Check sheet for the drawn part. Datum: minimum x, y, z corner. Units: mm. Give positions to 0.01 mm unless a question says otherwise; leave off trailing zeros. Loops run counter-clockwise (first coordinate to the right, second up) from the corner with the lowest first, then second, coordinate; pieces in that order, holes last. Notation, with made-up numbers: (-31.5, 0.25) - (-15.5, 0.25) arc R30 cw to (-15.5, 30.25) - close; hole circle Ø11 at (75, -24.75). An arc over 180 degrees is marked (long way). Use one line per item in the form item = value.
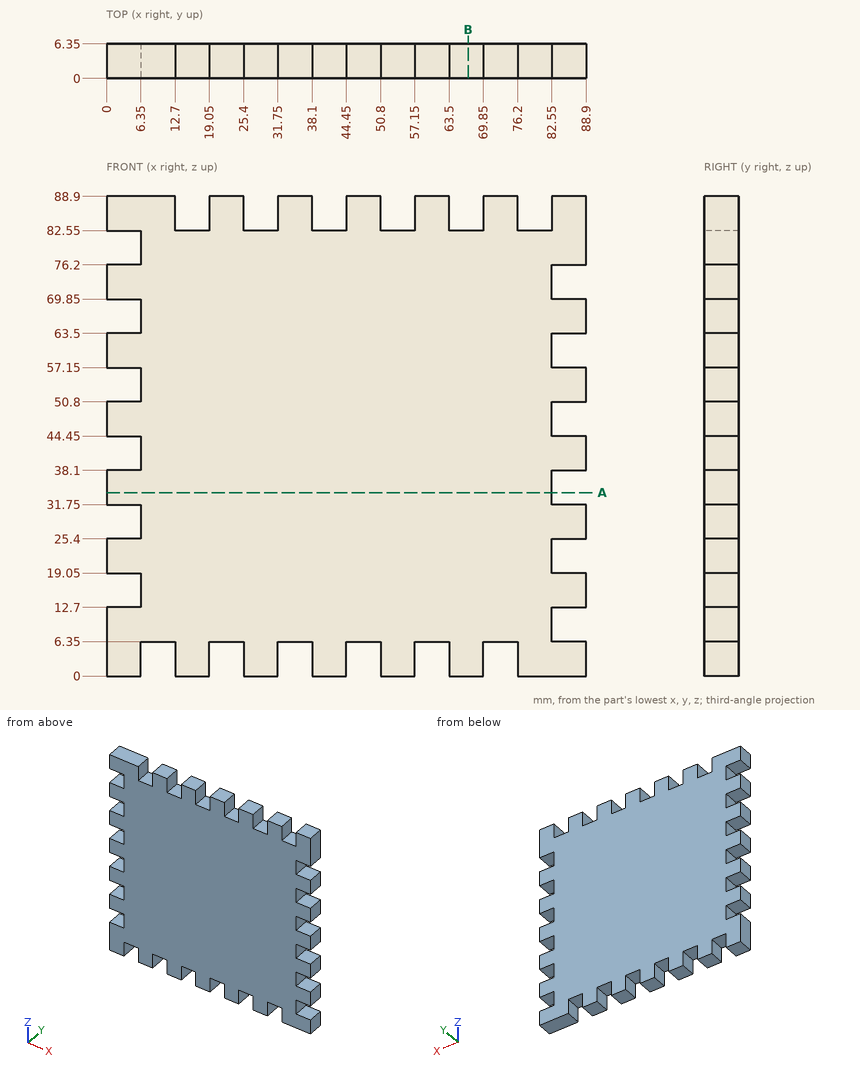
1. Scan lines: probe 1 along X at (y, z) = (4.5, 8); probe 2 along Z at (x, y) = (32.5, 4). Record each from-to range of solid material in increasing order.
Result set:
probe_1 = 0 to 82.55
probe_2 = 6.35 to 88.9
2. Section check A-A, the plane z = 34. Record the cut outline in (x, y).
Result set:
outline = (0, 0) - (82.55, 0) - (82.55, 6.35) - (0, 6.35) - close
3. Depth check by flat-ended pin: pin 1 Ø1 at (y, z) = (1.5, 50) entering from +X; pin 2 Ø1.9 at (y, z) = (3.5, 68) entering from -X; pin 3 Ø1.5 at (x, y) = (29.5, 5.5) entering from +Z. Enter the tip coordinate at first touch or a pass-through.
Result set:
pin_1 = 82.55
pin_2 = 6.35
pin_3 = 82.55
4. Section check B-B, the plane x = 67. Record the cut outline in (y, z), then the cut area to 3 significant figures.
Result set:
outline = (0, 0) - (6.35, 0) - (6.35, 82.55) - (0, 82.55) - close
area = 524 mm²
